Geometry check sheet. Reference: the model listing, model coordinates, mm. A direction names the side the tool comes from. Round coordinates to 2 decimals unless told otherwise and drop trailing zeros. Order: outer loops, then holes, each group sorted by start corner. A loop starts at its lowest first (then second) coordinate and runs counter-clockwise, first axis right, second up. Notation, with made-up numbers: (-39.5, 55.5) - (-34.5, 55.5) arc R19 ccw to (-34.5, 84.5) - close; hole circle Ø3 at (54.25, 73). An arc over 180 degrees is marked (long way). Return JSON: item names as keys, results as strings. Group by question number.
Q1. Gauge pin test, flat ends, axial feed: pin 1 Ø1 at (y, z) = (10.5, 2) entering from -X; pin 2 Ø2.5 at (x, y) = (19, -5) entering from +Z. Record the tip position at first contact, or that the pin passes through.
Q2. Tool access check on faces 1 (the flat face through (8, -20, 1)), 2 (the cylindrical face through (1.454, 15.465, 1.521)). Record the directions out of +Z, -Z, +X, -X, +Y, -Y that give a thin tool (end or side, any length) a straight path to the whole face; none if there is none.
Q3. Sectioned sample at D-D, the plane x = 5.75. Record the cut outline in (y, z).
Q4. Sectioned sample at B-B, the plane z = 2.5. Record the cut outline in (x, y), then the cut area to 3 significant figures.
Q5. Material ranges on line 1 along Y through (x, z) = (19, 1.45); line 2 along Y through (x, z) = (18, 1.8); line 3 along X through (y, z) = (-4, 1.7), recorded low to high.
Q6. Sectioned sample at C-C, the plane y = -5. Record the cut outline in (x, z), then the cut area to 3 significant figures.
Q7. Sectioned sample at A-A, the plane x = 19. Record the cut outline in (y, z).
Q8. Draft check along Y on faces 3 (the cylindrical face through (15, 0, 1)), 4 (the flat face through (11, 20, 1)), 5 (the flat face through (22, 4, 1)). Enter one of: pulls with the +Y half, pulls with the -Y half, needs draft (parallel to the pull), parting line crosses it, or undercut.
```python
from build123d import *

# Parameters (mm, degrees)
EXTRUDE_1_DEPTH     = 3
SKETCH_2_R          = 1.5
CUT_EXTRUDE_1_DEPTH = 30.883105595
FILLET_1_R          = 10
FILLET_2_R          = 2


with BuildPart() as part:
    # 草图1 → 凸台-拉伸1 (new body)
    with BuildSketch(Plane.XY):
        with BuildLine():
            Line((22, 20), (22, -20))
            Line((22, -20), (1, -20))
            Line((1, -20), (1, -14.966629547))
            ThreePointArc((1, -14.966629547), (15, 0), (1, 14.966629547))
            Line((1, 14.966629547), (1, 20))
            Line((1, 20), (22, 20))
        make_face()
    extrude(amount=EXTRUDE_1_DEPTH)

    # 草图2 → 切除-拉伸1 (cut, through all)
    with BuildSketch(Plane.XY.offset(3)):
        with Locations((19, 15)):
            Circle(SKETCH_2_R)
        with Locations((19, -5)):
            Circle(SKETCH_2_R)
    extrude(amount=-CUT_EXTRUDE_1_DEPTH, mode=Mode.SUBTRACT)

    # 圆角1
    fillet_1_edges = [part.edges().sort_by_distance(p)[0] for p in [
        (22, -20, 1.5),
    ]]
    fillet(fillet_1_edges, radius=FILLET_1_R)

    # 圆角2
    fillet_2_edges = [part.edges().sort_by_distance(p)[0] for p in [
        (1, 20, 1.5),
        (22, 20, 1.5),
        (1, -20, 1.5),
        (1, -14.966629547, 1.5),
        (1, 14.966629547, 1.5),
    ]]
    fillet(fillet_2_edges, radius=FILLET_2_R)


solid = part.part
```
Reply:
{
 "1": {"pin 1": "x = 10.2", "pin 2": "through"},
 "2": {"face 1": "+Z, -Z, +X, -X, -Y", "face 2": "+Z, -Z, -X"},
 "3": {"outline": "(-20, 0) - (-13.85, 0) - (-13.85, 3) - (-20, 3) - close; (13.85, 0) - (20, 0) - (20, 3) - (13.85, 3) - close"},
 "4": {"outline": "(1, -18) arc R2 ccw to (3, -20) - (12, -20) arc R10 ccw to (22, -10) - (22, 18) arc R2 ccw to (20, 20) - (3, 20) arc R2 ccw to (1, 18) - (1, 16.73) arc R2 ccw to (2.65, 14.76) arc R15 cw to (2.65, -14.76) arc R2 ccw to (1, -16.73) - close; hole circle Ø3 at (19, -5); hole circle Ø3 at (19, 15)", "area": "477 mm^2"},
 "5": {"line 1": "-17.14 to -6.5, -3.5 to 13.5, 16.5 to 20", "line 2": "-18 to -6.12, -3.88 to 13.88, 16.12 to 20", "line 3": "14.46 to 17.88, 20.12 to 22"},
 "6": {"outline": "(14.14, 0) - (17.5, 0) - (17.5, 3) - (14.14, 3) - close; (20.5, 0) - (22, 0) - (22, 3) - (20.5, 3) - close", "area": "14.6 mm^2"},
 "7": {"outline": "(-17.14, 0) - (-6.5, 0) - (-6.5, 3) - (-17.14, 3) - close; (-3.5, 0) - (13.5, 0) - (13.5, 3) - (-3.5, 3) - close; (16.5, 0) - (20, 0) - (20, 3) - (16.5, 3) - close"},
 "8": {"face 3": "undercut", "face 4": "pulls with the +Y half", "face 5": "needs draft"}
}
